```python
from build123d import *

# Parameters (mm, degrees)
F1_DEPTH      = 2
F1_DEPTH_BACK = 2
F3_DEPTH      = 2.5
F3_DEPTH_BACK = 2.5
F5_DEPTH      = 3


with BuildPart() as f1:
    # F0 (on Top) → F1 (new body, two sides)
    with BuildSketch(Plane.XY) as f1_sk:
        with BuildLine():
            Line((14.011182, 2.911577), (19, 6.244998))
            ThreePointArc((19, 6.244998), (0, 20), (-19, 6.244998))
            Line((-19, 6.244998), (-14.011182, 2.911577))
            Line((-14.011182, 2.911577), (-14.011182, -1.588423))
            Line((-14.011182, -1.588423), (-3.011182, -1.588423))
            Line((-3.011182, -1.588423), (-3.011182, 14.988818))
            ThreePointArc((-3.011182, 14.988818), (-2.129227, 17.118045), (0, 18))
            ThreePointArc((0, 18), (2.129227, 17.118045), (3.011182, 14.988818))
            Line((3.011182, 14.988818), (3.011182, -1.588423))
            Line((3.011182, -1.588423), (14.011182, -1.588423))
            Line((14.011182, -1.588423), (14.011182, 2.911577))
        make_face()
    extrude(amount=F1_DEPTH)
    extrude(f1_sk.sketch, amount=-F1_DEPTH_BACK)

    # F2 (on Top) → F3 (join, two sides)
    with BuildSketch(Plane.XY) as f3_sk:
        with BuildLine():
            Line((19.186818, 5.644998), (20.055932, 6.225721))
            ThreePointArc((20.055932, 6.225721), (0, 21), (-20.055932, 6.225721))
            Line((-20.055932, 6.225721), (-19.186818, 5.644998))
            ThreePointArc((-19.186818, 5.644998), (0, 20), (19.186818, 5.644998))
        make_face()
    extrude(amount=F3_DEPTH)
    extrude(f3_sk.sketch, amount=-F3_DEPTH_BACK)

    # F4 (on face) → F5 (cut)
    with BuildSketch(Plane.XY.offset(2)):
        with BuildLine():
            Line((-11.011182, 4.411577), (-11.011182, -1.588423))
            Line((-11.011182, -1.588423), (-6.011182, -1.588423))
            Line((-6.011182, -1.588423), (-6.011182, 4.411577))
            ThreePointArc((-6.011182, 4.411577), (-8.511182, 6.911577), (-11.011182, 4.411577))
        make_face()
        with BuildLine():
            Line((6.011182, 4.411577), (6.011182, -1.588423))
            Line((6.011182, -1.588423), (11.011182, -1.588423))
            Line((11.011182, -1.588423), (11.011182, 4.411577))
            ThreePointArc((11.011182, 4.411577), (8.511182, 6.911577), (6.011182, 4.411577))
        make_face()
    extrude(amount=-F5_DEPTH, mode=Mode.SUBTRACT)


solid = f1.part
```
Source: CAD feature listing. Evaluate the final solid. Frame: model axes, mm. A direction names the side the tool comes from. Round coordinates to 2 decimals unless told otherwise and drop trailing zeros. Loops run counter-clockwise (first coordinate to the right, second up) from the corner with the lowest first, then second, coordinate; pieces in that order, holes last.
1. Section query C-C on x = -3.5. Output: boundary loops of the cut face in (y, z).
2. Section query A-A on y = 5. Output: boundary loops of the cut face in (x, z).
3. Section query B-B on z = 1.4. Output: boundary loops of the cut face in (x, y) (3 decimals), and give its area (3 significant figures).
4. Ray query, L1, parallel to X at y = 1.25, z = -0.75; L2, parallel to X at y = 3.75, z = 1.15; L3, parallel to Z at x = 6, y = 11.5. Return the intervals inside material, ascending.
5. Contact query for flat-ended pins moving along their axis: pin 1 (0.9 mm diameter, centred on y = 1.5, z = 0.5, fed in from +X); pin 2 (2.5 mm diameter, centred on x = -8, y = 5, fed in from +Z); pin 3 (3 mm diameter, centred on x = -8, z = 0, fed in from -Y); pin 4 (6.5 mm diameter, centred on x = -6.5, y = 4, fed in from -Z). Output: stop coordinate, or through.
6. Access query for faces 1 (the flat face through (16.471, 4.555, 0.028)), 2 (the flat face through (6.011, 1, 1)), 3 (the flat face through (14.011, 1, 0)). Directions: +Z, -Z, +X, -X, +Y, -Y. A direction counts if a zero-diameter tool reaches every point of the face in a straight line with its end or side. Return the directions, or none.
7. Section query D-D on y = 13.75. Output: boundary loops of the cut face in (x, z).
Answers below:
1. outline: (-1.59, -2) - (19.69, -2) - (19.69, -2.5) - (20.71, -2.5) - (20.71, 2.5) - (19.69, 2.5) - (19.69, 2) - (-1.59, 2) - close
2. outline: (-17.14, -2) - (-3.01, -2) - (-3.01, 2) - (-6.08, 2) - (-6.08, -1) - (-10.94, -1) - (-10.94, 2) - (-17.14, 2) - close; (3.01, -2) - (17.14, -2) - (17.14, 2) - (10.94, 2) - (10.94, -1) - (6.08, -1) - (6.08, 2) - (3.01, 2) - close
3. outline: (-20.056, 6.226) - (-19.187, 5.645) arc R20 cw to (-19, 6.245) - (-14.011, 2.912) - (-14.011, -1.588) - (-11.011, -1.588) - (-11.011, 4.412) arc R2.5 cw to (-6.011, 4.412) - (-6.011, -1.588) - (-3.011, -1.588) - (-3.011, 14.989) arc R3.011 cw to (0, 18) arc R3.011 cw to (3.011, 14.989) - (3.011, -1.588) - (6.011, -1.588) - (6.011, 4.412) arc R2.5 cw to (11.011, 4.412) - (11.011, -1.588) - (14.011, -1.588) - (14.011, 2.912) - (19, 6.245) arc R20 cw to (19.187, 5.645) - (20.056, 6.226) arc R21 ccw to start
3. area: 477 mm2
4. L1: x = -14.01 to -11.01, -6.01 to -3.01, 3.01 to 6.01, 11.01 to 14.01
4. L2: x = -15.27 to -11.01, -6.01 to -3.01, 3.01 to 6.01, 11.01 to 15.27
4. L3: z = -2 to 2
5. pin 1: stops at x = 14.01
5. pin 2: stops at z = -1
5. pin 3: stops at y = -1.59
5. pin 4: stops at z = -2
6. face 1: +Z, -Z, -Y
6. face 2: +Z, -Y
6. face 3: +Z, -Z, +X, -Y
7. outline: (-15.87, -2.5) - (-14.52, -2.5) - (-14.52, -2) - (-3.01, -2) - (-3.01, 2) - (-14.52, 2) - (-14.52, 2.5) - (-15.87, 2.5) - close; (3.01, -2) - (14.52, -2) - (14.52, -2.5) - (15.87, -2.5) - (15.87, 2.5) - (14.52, 2.5) - (14.52, 2) - (3.01, 2) - close
